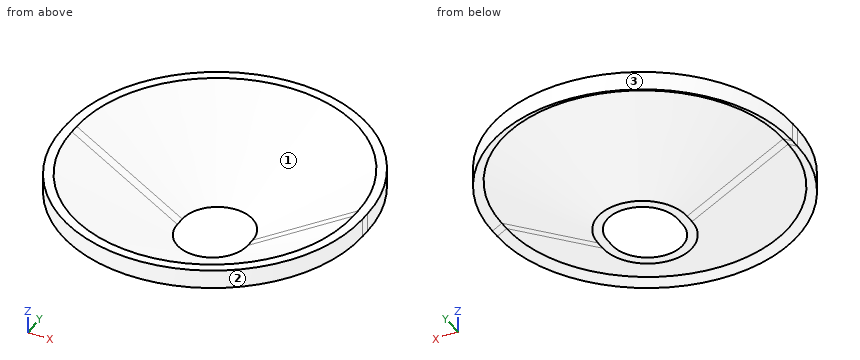
```python
from build123d import *


with BuildPart() as f2:
    # F2: sweep along a path in F0
    with BuildLine(Plane.XY) as f2_path:
        ThreePointArc((4.75, 0.5), (0, 5.25), (-4.75, 0.5))
        Line((-4.75, 0.5), (-4.75, -0.5))
        ThreePointArc((-4.75, -0.5), (0, -5.25), (4.75, -0.5))
        Line((4.75, -0.5), (4.75, 0.5))
    # F1 (on Front) → F2 (sweep)
    with BuildSketch(Plane.XZ):
        Polygon((3.75, 0), (4.75, 0), (15, 5.57735), (16, 5), (16, 7), (15, 7), align=None)
    sweep(path=f2_path.line)


solid = f2.part
```
Work out the finished part from the listing and answer in its coordinate system (mm). Face numbers are marked on the shaded views. Give positions to 0.01 mm unless a question says otherwise; leave off trailing zeros. Write each loop counter-clockwise with the first axis right and the second up, starting at its lowest first coordinate (ties: lowest second). Pieces come first, ordered by that corner, then holes. Notation, with made-up numbers: (27.25, -12.75) -> (64.25, -12.75) arc R25 ccw to (64.25, 11.25) -> close; hole circle Ø1 at (-34.75, -34.75). An arc over 180 degrees is marked (long way). Write each question's results on one line, items separated by ' | '.
1. Each of these flat-tipped pins is pushed along its axis until it touches: pin 1 Ø4 at (y, z) = (-4.5, 6) entering from -X; pin 2 Ø10 at (x, y) = (-3.5, 4.5) entering from +Z; pin 3 Ø12 at (x, y) = (0.5, -3) entering from +Z. Where does it stop, or does it pass through?
Data:
pin 1: x = -15.87 | pin 2: z = 4.08 | pin 3: z = 2.99
2. Find section B-B on z = 3.75. Determine the outline of the cut face in (x, y).
Data:
outline: (-11.64, -0.5) arc R11.64 ccw to (11.64, -0.5) -> (11.64, 0.5) arc R11.64 ccw to (-11.64, 0.5) -> close; hole (-9.78, -0.5) arc R9.78 ccw to (9.78, -0.5) -> (9.78, 0.5) arc R9.78 ccw to (-9.78, 0.5) -> close
3. Straight lines are drawn through the part: L1, parallel to X at y = -3, z = 5.5; L2, parallel to Y at x = -1, z = 3.25; L3, parallel to Y at x = -4.5, z = 5.25. For each, find the intervals that lie inside material, in ascending order.
Data:
L1: -15.8 to -14.93, -14.65 to -12.34, 12.34 to 14.65, 14.93 to 15.8 | L2: -11.18 to -9.42, 9.42 to 11.18 | L3: -15.85 to -15.4, -14.18 to -11.83, 11.83 to 14.18, 15.4 to 15.85
4. Find section A-A on x = 0. Determine the outline of the cut face in (y, z).
Data:
outline: (-16.5, 5) -> (-15.5, 5.58) -> (-5.25, 0) -> (-4.25, 0) -> (-15.5, 7) -> (-16.5, 7) -> close; (4.25, 0) -> (5.25, 0) -> (15.5, 5.58) -> (16.5, 5) -> (16.5, 7) -> (15.5, 7) -> close
5. Determine the mould class of the marked faces 1, 2 and 3 for opening direction Y: +Y half, -Y half, draft (parallel to the pull), parting line (faces both ways), or undercut.
Data:
face 1: undercut | face 2: -Y half | face 3: +Y half
6. Find section C-C on z = 6. Determine the outline of the cut face in (x, y).
Data:
outline: (-16, -0.5) arc R16 ccw to (16, -0.5) -> (16, 0.5) arc R16 ccw to (-16, 0.5) -> close; hole (-13.39, -0.5) arc R13.39 ccw to (13.39, -0.5) -> (13.39, 0.5) arc R13.39 ccw to (-13.39, 0.5) -> close
